from build123d import *

# Parameters (mm, degrees)
SKETCH2_W               = 50.634745493
SKETCH2_H               = 13.07277583
CUT_EXTRUDE1_DEPTH      = 5.0000001
CUT_EXTRUDE1_DEPTH_BACK = 5.0000001
SKETCH3_R               = 1
CUT_EXTRUDE2_DEPTH      = 5.0000001
SKETCH4_R               = 2.1
CUT_EXTRUDE3_DEPTH      = 4.0000001
CUT_EXTRUDE5_DEPTH      = 5.0000001


with BuildPart() as part:
    # Sketch1 → Revolve1 (revolve)
    with BuildSketch(Plane.XY):
        with BuildLine():
            Line((-14, 0), (14, 0))
            add(Edge.make_bspline(
                [(14, 0), (14, 4), (0, 4), (-14, 4), (-14, 0)],
                knots=[0, 0, 0, 1.570796327, 1.570796327, 3.141592654, 3.141592654, 3.141592654], degree=2, weights=[1, 0.707106781, 1, 0.707106781, 1]))
        make_face()
    revolve(axis=Axis((-14, 0, 0), (1, 0, 0)))

    # Sketch2 → Cut-Extrude1 (cut, two sides)
    with BuildSketch(Plane.XY) as cut_extrude1_sk:
        with Locations((-1.598405816, -6.536387915)):
            Rectangle(SKETCH2_W, SKETCH2_H)
    extrude(amount=CUT_EXTRUDE1_DEPTH, mode=Mode.SUBTRACT)
    extrude(cut_extrude1_sk.sketch, amount=-CUT_EXTRUDE1_DEPTH_BACK, mode=Mode.SUBTRACT)

    # Sketch3 → Cut-Extrude2 (cut, through all)
    with BuildSketch(Plane.XZ):
        with Locations((-12, 0)):
            Circle(SKETCH3_R)
        with Locations((3, 0)):
            Circle(SKETCH3_R)
    extrude(amount=-CUT_EXTRUDE2_DEPTH, mode=Mode.SUBTRACT)

    # Sketch4 → Cut-Extrude3 (cut, through all)
    with BuildSketch(Plane(origin=(0, 1, 0), x_dir=(-1, 0, 0), z_dir=(0, -1, 0))):
        with Locations((12, 0)):
            Circle(SKETCH4_R)
        with Locations((-3, 0)):
            Circle(SKETCH4_R)
    extrude(amount=-CUT_EXTRUDE3_DEPTH, mode=Mode.SUBTRACT)

    # Sketch6 → Cut-Extrude5 (cut, through all)
    with BuildSketch(Plane.XZ):
        with BuildLine():
            Line((4.406700976, 3.796679392), (7.593299024, -3.360537007))
            add(Edge.make_bspline(
                [(7.593299024, -3.360537007), (14, -2.178801768), (14, 0)],
                knots=[5.285654608, 5.285654608, 5.285654608, 6.283185307, 6.283185307, 6.283185307], degree=2, weights=[1, 0.878173816, 1]))
            add(Edge.make_bspline(
                [(14, 0), (14, 2.887726136), (4.406700976, 3.796679392)],
                knots=[0, 0, 0, 1.250587947, 1.250587947, 1.250587947], degree=2, weights=[1, 0.810791081, 1]))
        make_face()
    extrude(amount=-CUT_EXTRUDE5_DEPTH, mode=Mode.SUBTRACT)


solid = part.part
Check sheet for the modelled part. Datum: model origin and axes. Units: mm. A direction names the side the tool comes from. Round coordinates to 2 decimals unless told otherwise and drop trailing zeros.
(1) Scan lines: probe 1 along Z at (x, y) = (-12, 0.4); probe 2 along Z at (x, y) = (3.25, 2.7); probe 3 along Y at (x, z) = (-3, -1.5). Record each from-to range of solid material in increasing order.
(2) Go/stop test with flat-tipped pins: P1, Ø4, axis at x = -12.5, z = 0, coming from the +Y side; P2, Ø1.6, axis at x = 3, z = 0, coming from the +Y side; P3, Ø1, axis at x = -2, z = 2.5, coming from the +Y side; P4, Ø2, axis at x = -3, z = -0.5, coming from the +Y side. Record where each tip stops, or that it passes through.
(3) Access from +Z, -Z, +X, -X, +Y, -Y to the whole of each face (thin tool, end or side, straight path). Record for faces 4 (the cylindrical face through (-13, 0.5, 0)), 5 (the flat face through (-10.9, 1, 0.4)).
(4) Draft check along X on faces 1 (the cylindrical face through (-9.9, 1.7, 0)), 2 (the flat face through (5.978, 1.378, 0.268)), 3 (the cylindrical face through (0.997, 2.475, -0.631)). Enter one of: pulls with the +X half, pulls with the -X half, needs draft (parallel to the pull), parting line crosses it, or undercut.
(5) Cross-section at A-A, the plane z = 0. State how many separate pieces and enclosed holes the cut face has, and give its area (3 significant figures).
Check sheet entries:
1. probe 1: z = -2.02 to -1, 1 to 2.02
1. probe 2: z = -2.8 to -2.09, 2.09 to 2.8
1. probe 3: y = 0 to 3.61
2. P1: stops at y = 1
2. P2: passes through
2. P3: stops at y = 3.42
2. P4: stops at y = 3.95
3. face 4: +Y, -Y
3. face 5: -X, +Y
4. face 1: pulls with the -X half
4. face 2: pulls with the +X half
4. face 3: undercut
5. separate pieces: 3
5. enclosed holes: 0
5. area: 47.4 mm2
